Can you work these out from the model? Positions are in its coordinate system, mm. A direction names the side the tool comes from. Give positions to 0.01 mm unless a question says otherwise; leave off trailing zeros. Write each loop counter-clockwise with the first axis right and the second up, starting at its lowest first coordinate (ties: lowest second). Pieces come first, ordered by that corner, then holes. Notation, with made-up numbers: (45, 37) - (96, 37) arc R31 cw to (96, 71) - close; hole circle Ø6 at (-6.5, 65). An arc over 180 degrees is marked (long way). Use a Markdown table: item, result. Add a question column.
```python
from build123d import *

# Parameters (mm, degrees)
SKIZZE1_W                       = 39.5
SKIZZE1_H                       = 39
AUFSATZ_LINEAR_AUSTRAGEN1_DEPTH = 2
F_3_0_3_DURCHMESSER_BOHRUNG1_D  = 3
SKIZZE4_W                       = 1
SKIZZE4_H                       = 39
SCHNITT_LINEAR_AUSTRAGEN1_DEPTH = 0.5
VERRUNDUNG1_R                   = 1


with BuildPart() as part:
    # Skizze1 → Aufsatz-Linear austragen1 (new body)
    with BuildSketch(Plane(origin=(0, 0, 0), x_dir=(1, 0, 0), z_dir=(0, 1, 0))):
        with Locations((19.75, -19.5)):
            Rectangle(SKIZZE1_W, SKIZZE1_H)
    extrude(amount=AUFSATZ_LINEAR_AUSTRAGEN1_DEPTH)

    # Ø3.0 (3) Durchmesser Bohrung1 (through all)
    with Locations(Plane(origin=(0, 2, 0), x_dir=(1, 0, 0), z_dir=(0, 1, 0))):
        with Locations((36.5, -3), (36.5, -36)):
            Hole(F_3_0_3_DURCHMESSER_BOHRUNG1_D / 2)

    # Skizze4 → Schnitt-Linear austragen1 (cut)
    with BuildSketch(Plane(origin=(0, 2, 0), x_dir=(1, 0, 0), z_dir=(0, 1, 0))):
        with Locations((0.5, -19.5)):
            Rectangle(SKIZZE4_W, SKIZZE4_H)
    extrude(amount=-SCHNITT_LINEAR_AUSTRAGEN1_DEPTH, mode=Mode.SUBTRACT)

    # Verrundung1
    verrundung1_edges = [part.edges().sort_by_distance(p)[0] for p in [
        (0, 0.75, 0),
        (0, 0.75, 39),
    ]]
    fillet(verrundung1_edges, radius=VERRUNDUNG1_R)


solid = part.part
```
Q1. Suppose I cut it at A-A (x = 36.5). Please give me the cut outline in (y, z), and give its area (3 significant figures).
Q2. If we mould it in two halves opening along Z, with no side actions, what happens to faces 3 (the cylindrical face through (38, 1, 3)), 4 (the flat face through (0, 1, 20)), 5 (the cylindrical face through (37.7, 1, 36.9)), 6 (the cylindrical face through (0.285, 0.76, 0.301))? For each: released by +Z, released by -Z, zero draft, split by the parting line, or undercut.
Q3. If I drill on probe 1 along Z at (x, y) = (36.5, 1); probe 2 along Z at (x, y) = (37, 1.8); probe 3 along X at (y, z) = (0.2, 4), over which ranges is the centre line in solid material (lowest first)? Write a range as [from, to].
Q4. Suppose I cut it at B-B (z = 36). Please give me the cut outline in (x, y).
Q5. On a 3-axis mill with a long thin cutter (end or side, diameter ignored), from which of +Z, -Z, +X, -X, +Y, -Y can I reach the whole of each face in a straight line? I mean faces 1 (the flat face through (20, 1, 39)), 2 (the flat face through (0.5, 1.5, 19.2)). Say none if no direction works.
Q6. I'm going to push flat-ended pins straight in: P1, Ø0.8, axis at x = 0.5, z = 19, coming from the +Y side; P2, Ø0.6, axis at y = 2, z = 23.5, coming from the -X side; P3, Ø2.5, axis at x = 36.5, z = 36, coming from the +Y side. Where does each tip first touch, or does it pass through?
Derived:
| question | item | result |
|---|---|---|
| 1 | outline | (0, 0) - (2, 0) - (2, 1.5) - (0, 1.5) - close; (0, 4.5) - (2, 4.5) - (2, 34.5) - (0, 34.5) - close; (0, 37.5) - (2, 37.5) - (2, 39) - (0, 39) - close |
| 1 | area | 66.0 mm² |
| 2 | face 3 | undercut |
| 2 | face 4 | zero draft |
| 2 | face 5 | undercut |
| 2 | face 6 | released by -Z |
| 3 | probe 1 | [0, 1.5], [4.5, 34.5], [37.5, 39] |
| 3 | probe 2 | [0, 1.59], [4.41, 34.59], [37.41, 39] |
| 3 | probe 3 | [0, 35.38], [37.62, 39.5] |
| 4 | outline | (0, 0) - (35, 0) - (35, 2) - (1, 2) - (1, 1.5) - (0, 1.5) - close; (38, 0) - (39.5, 0) - (39.5, 2) - (38, 2) - close |
| 5 | face 1 | +Z, +X, -X, +Y, -Y |
| 5 | face 2 | +Z, -Z, -X, +Y |
| 6 | P1 | y = 1.5 |
| 6 | P2 | x = 1 |
| 6 | P3 | through |
